Study the drawing (mm; zero at the part's minimum x, y, z) and answer. Round coordinates to 2 decimals unless told otherwise and drop trailing zeros. Order: outer loops, then holes, each group sorted by start corner. A loop starts at its lowest first (then second) coordinate and runs counter-clockwise, first axis right, second up. Notation, with made-up numbers: (-10.5, 39) - (48.5, 39) arc R18 ccw to (48.5, 49) - close; hole circle Ø6 at (-39.75, -39.5). An arc over 180 degrees is marked (long way). Put each result on its own line as item: value. Start each with the question number.
Q1. Section D-D on z = 57 is taken. Give the vertices of the cut face in (x, y).
Q2. Section C-C on y = 2.8 is taken. State how many separate pieces and enclosed holes the cut face has, then the cut area to 3 significant figures.
Q3. Section A-A on x = 53 is taken. Give the vertices of the cut face in (y, z).
Q4. For a pull along X with two mould halves and no side action, classify the marked faces 1 and 2 as pulls with the +X half, pulls with the -X half, needs draft (parallel to the pull), parting line crosses it, or undercut.
Q5. Each of these flat-tipped pins is pushed along its axis until it touches: pin 1 Ø1.6 at (y, z) = (3, 38.5) entering from -X; pin 2 Ø0.6 at (x, y) = (120.5, 2.5) entering from +Z; pin 3 Ø1 at (y, z) = (3, 31) entering from +X; pin 4 Ø1.5 at (x, y) = (224, 3.5) entering from +Z. Where does it stop, or does it pass through?
Q6. Section B-B on z = 73.5 is taken. Give the vertices of the cut face in (x, y).
Q7. Find the intervals of material crossed by line 1 along X through (y, z) = (3.35, 46.5); line 2 along X through (y, z) = (2.75, 69); line 3 along Y through (x, z) = (224, 64), in increasing order. Write a range as from..to.
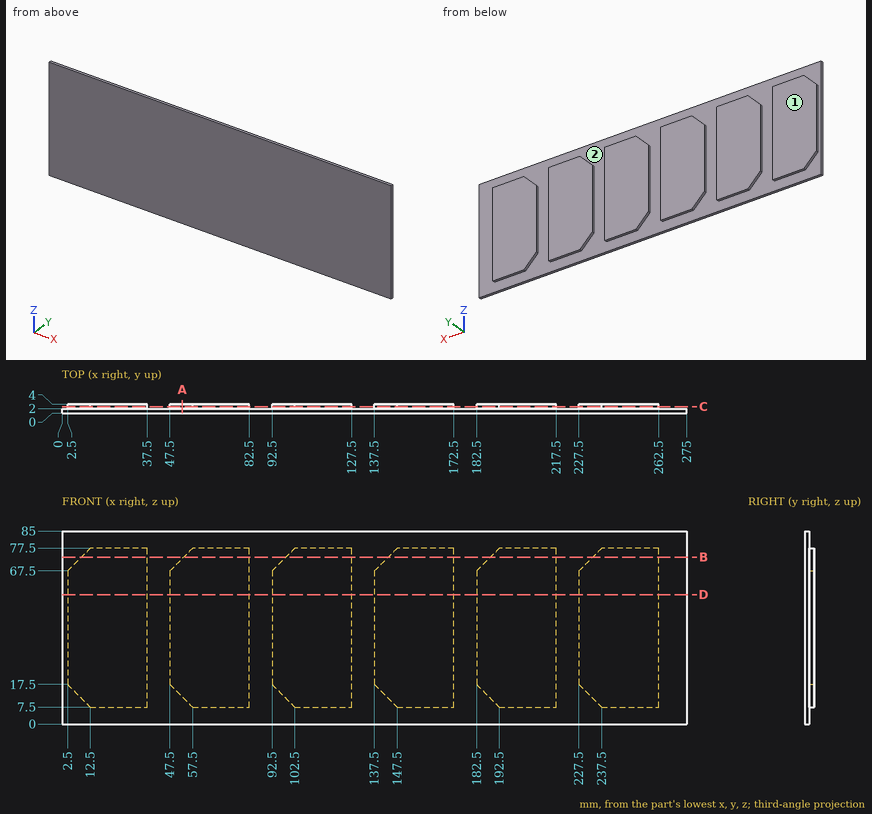
Findings:
1. outline: (0, 0) - (275, 0) - (275, 2) - (262.5, 2) - (262.5, 4) - (227.5, 4) - (227.5, 2) - (217.5, 2) - (217.5, 4) - (182.5, 4) - (182.5, 2) - (172.5, 2) - (172.5, 4) - (137.5, 4) - (137.5, 2) - (127.5, 2) - (127.5, 4) - (92.5, 4) - (92.5, 2) - (82.5, 2) - (82.5, 4) - (47.5, 4) - (47.5, 2) - (37.5, 2) - (37.5, 4) - (2.5, 4) - (2.5, 2) - (0, 2) - close
2. separate pieces: 6
2. enclosed holes: 0
2. area: 14,100 mm2
3. outline: (0, 0) - (2, 0) - (2, 12) - (4, 12) - (4, 73) - (2, 73) - (2, 85) - (0, 85) - close
4. face 1: needs draft
4. face 2: undercut
5. pin 1: x = 2.5
5. pin 2: z = 77.5
5. pin 3: x = 262.5
5. pin 4: through
6. outline: (0, 0) - (275, 0) - (275, 2) - (262.5, 2) - (262.5, 4) - (233.5, 4) - (233.5, 2) - (217.5, 2) - (217.5, 4) - (188.5, 4) - (188.5, 2) - (172.5, 2) - (172.5, 4) - (143.5, 4) - (143.5, 2) - (127.5, 2) - (127.5, 4) - (98.5, 4) - (98.5, 2) - (82.5, 2) - (82.5, 4) - (53.5, 4) - (53.5, 2) - (37.5, 2) - (37.5, 4) - (8.5, 4) - (8.5, 2) - (0, 2) - close
7. line 1: 2.5..37.5, 47.5..82.5, 92.5..127.5, 137.5..172.5, 182.5..217.5, 227.5..262.5
7. line 2: 4..37.5, 49..82.5, 94..127.5, 139..172.5, 184..217.5, 229..262.5
7. line 3: 0..2
